Design review of the part built by this model. Coordinates are the model's own, in mm. Give positions to 0.01 mm unless a question says otherwise; leave off trailing zeros. Write each loop counter-clockwise with the first axis right and the second up, starting at its lowest first coordinate (ties: lowest second). Pieces come first, ordered by that corner, then holes. Notation, with made-up numbers: M 3,49 L 44,49 A17 ccw 44,80 Z; hole C 14,12 d1. An arc over 180 degrees is marked long. Answer in a Markdown table with one row per item.
Autodesk Inventor part; units mm, degrees
ref_plane "YZ Plane" through (0, 0, 0) normal (1, 0, 0) x (0, 1, 0)
ref_plane "XZ Plane" through (0, 0, 0) normal (0, 1, 0) x (-1, 0, 0)
ref_plane "XY Plane" through (0, 0, 0) normal (0, 0, 1) x (1, 0, 0)
sketch "Boceto1" plane through (0, 0, 0) normal (0, 1, 0) x (-1, 0, 0)
  circle A0 centre (0, 0) radius 60
  circle A1 centre (0, 0) radius 50
  line L0 (0, 0) -> (0, -60)
  line L1 (0, -60) -> (0, -50)
  circle A2 centre (0, -55) radius 1.15
  dimension "d0" = 120
  dimension "d1" = 100
  dimension "d2" = 2.3
extrude "Extrusión1" add sketch "Boceto1" along normal blind 2 contours A2 L0 | L0 A2 | A0
sketch "Boceto2" plane through (0, 2, 0) normal (0, 1, 0) x (1, 0, 0)
  circle A0 centre (0, 0) radius 50
  line L0 (0, 50) -> (0, 60)
  circle A1 centre (0, 0) radius 60
  circle A2 centre (0, 55) radius 1.15
  circle A3 centre (-55, 0) radius 1.15
  circle A4 centre (0, -55) radius 1.15
  circle A5 centre (55, 0) radius 1.15
  dimension "d5" = 2.3
  dimension "d8" = 360
extrude "Extrusión2" add sketch "Boceto2" along normal blind 2 contours A2 L0 | L0 A2 | A3 | A4 | A5
sketch "Boceto3" plane through (0, 0, 0) normal (0, -1, 0) x (1, 0, 0)
  circle A0 centre (0, 0) radius 50
  line L0 (-50, 0) -> (50, 0)
  arc A1 (-50.04, -1.9996) -> (-49.96, -1.9996) centre (-50, 0) ccw
  line L1 (-50.04, -1.9996) -> (-49.96, -1.9996)
  line L2 (-49.96, -1.9996) -> (-52.96, -1.9996)
  line L3 (-52.96, -1.9996) -> (-52.96, 2.2646)
  line L4 (-49.96, 1.9996) -> (-52.96, 2.0596)
  circle A2 centre (0, 0) radius 50
  line L5 (-28.2117, 44.8649) -> (-24.5188, 46.997)
  line L6 (-23.2483, 44.2664) -> (-24.6963, 46.8945)
  line L7 (-26.7117, 42.2668) -> (-28.2117, 44.8649)
  line L8 (24.7483, 46.8645) -> (28.4412, 44.7324)
  line L9 (26.7117, 42.2668) -> (28.2637, 44.8349)
  line L10 (23.2483, 44.2664) -> (24.7483, 46.8645)
  line L11 (52.96, 1.9996) -> (52.96, -2.2646)
  line L12 (49.96, -1.9996) -> (52.96, -2.0596)
  line L13 (49.96, 1.9996) -> (52.96, 1.9996)
  line L14 (28.2117, -44.8649) -> (24.5188, -46.997)
  line L15 (23.2483, -44.2664) -> (24.6963, -46.8945)
  line L16 (26.7117, -42.2668) -> (28.2117, -44.8649)
  line L17 (-24.7483, -46.8645) -> (-28.4412, -44.7324)
  line L18 (-26.7117, -42.2668) -> (-28.2637, -44.8349)
  line L19 (-23.2483, -44.2664) -> (-24.7483, -46.8645)
  line L20 (1.9996, -49.96) -> (1.9996, -52.96)
  line L21 (1.9996, -52.96) -> (-2.2646, -52.96)
  line L22 (-1.9996, -49.96) -> (-2.0596, -52.96)
  line L23 (49.96, 1.9996) -> (52.96, 1.9996)
  line L24 (52.96, 1.9996) -> (52.96, -2.2646)
  line L25 (49.96, -1.9996) -> (52.96, -2.0596)
  line L26 (-1.9996, 49.96) -> (-1.9996, 52.96)
  line L27 (-1.9996, 52.96) -> (2.2646, 52.96)
  line L28 (1.9996, 49.96) -> (2.0596, 52.96)
  point P0 (-52.96, 1.9996)
  point P1 (-24.7483, 46.8645)
  point P2 (-26.7517, 42.3361)
  point P3 (28.2117, 44.8649)
  point P4 (23.2883, 44.3357)
  point P5 (52.96, -1.9996)
  point P6 (50.04, 1.9996)
  point P7 (24.7483, -46.8645)
  point P8 (26.7517, -42.3361)
  point P9 (-28.2117, -44.8649)
  point P10 (-23.2883, -44.3357)
  point P11 (1.9996, -50.04)
  point P12 (-1.9996, -52.96)
  point P13 (50.04, 1.9996)
  point P14 (52.96, -1.9996)
  point P15 (-1.9996, 50.04)
  point P16 (1.9996, 52.96)
  dimension "d13" = 3
  dimension "d14" = 100
  dimension "d17" = 360
  dimension "d21" = 360
extrude "Extrusión3" add sketch "Boceto3" along normal blind 2 contours A0 L13 L11 L12 | A0 A1 L2 L3 L4 | A0 L26 L27 L28 | L20 L21 L22 A0
properties part number "ayudasoporte"
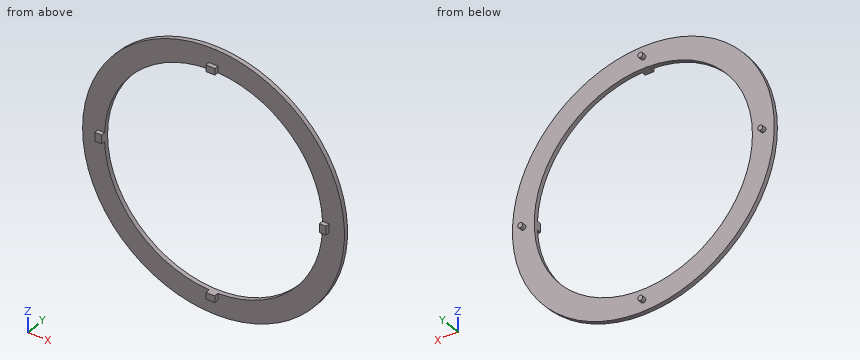
1) Add section A-A (z = 37.5). Write out the cut boundary in (x, y), and give its area (3 significant figures).
Geometry says:
| item | result |
|---|---|
| outline | M -46.84,0 L -33.07,0 L -33.07,2 L -46.84,2 Z; M 33.07,0 L 46.84,0 L 46.84,2 L 33.07,2 Z |
| area | 55.1 mm^2 |
2) Insertion check: P1, Ø1.6, axis at x = -52, y = -1, coming from the -Z side; P2, Ø2, axis at y = -0.5, z = -25, coming from the -X side; P3, Ø1, axis at y = 2, z = 39.5, coming from the +X side. Each pin has a flat end and moves straight along its axis. Give the tip position at first contact, or say it passes through.
Geometry says:
| item | result |
|---|---|
| P1 | z = -2 |
| P2 | x = -54.93 |
| P3 | x = 45.6 |
3) Add section C-C (y = 1.05). Write out the cut boundary in (x, z).
Geometry says:
| item | result |
|---|---|
| outline | C 0,0 d120; hole C 0,0 d100 |
4) Add section B-B (x = -34). Write out the cut boundary in (y, z), and give its area (3 significant figures).
Geometry says:
| item | result |
|---|---|
| outline | M 0,-49.44 L 2,-49.44 L 2,-36.66 L 0,-36.66 Z; M 0,36.66 L 2,36.66 L 2,49.44 L 0,49.44 Z |
| area | 51.1 mm^2 |
5) To check wall thickness, follow probe 1 along Z at (x, y) = (0, 0.05); probe 2 along X at (y, z) = (-0.75, 0). State the ranges of each line that lie inside material, in increasing order. Write a range as [from, to].
Geometry says:
| item | result |
|---|---|
| probe 1 | [-60, -50], [50, 60] |
| probe 2 | [-52.96, -50], [50, 52.96] |
